Autodesk Inventor part; units mm, degrees
ref_plane "ROD_BA_XY" through (8, 0, 0) normal (-1, 0, 0) x (0, 0, -1)
ref_plane "ROD_BA_YZ" through (8, 0, 0) normal (0, 0, -1) x (0, -1, 0)
ref_plane "ROD_BA_ZX" through (8, 0, 0) normal (0, -1, 0) x (-1, 0, 0)
sketch "Sketch_2" plane through (0, 0, 0) normal (0, 0, 1) x (1, 0, 0)
  line L0 (75.5, 0) -> (0, 0)
  line L1 (0, 0) -> (0, 1.5705)
  line L2 (0, 1.5705) -> (0.4295, 2)
  line L3 (0.4295, 2) -> (15, 2)
  line L4 (15, 2) -> (15, 1.65)
  line L5 (15, 1.65) -> (16.5, 1.65)
  line L6 (16.5, 1.65) -> (16.5, 2)
  line L7 (16.5, 2) -> (70.5, 2)
  line L8 (70.5, 2) -> (70.5, 5)
  line L9 (70.5, 5) -> (75.5, 5)
  line L10 (75.5, 5) -> (75.5, 0)
  line L11 (75.5, 0) -> (0, 0)
revolve "Revolution1" add sketch "Sketch_2" angle 360 about axis through (75.5, 0, 0) along (1, 0, 0)
thread "Thread1"
ref_plane "ROD_BA_XY" through (8, 0, 0) normal (-1, 0, 0) x (0, 0, -1)
ref_plane "ROD_BA_YZ" through (8, 0, 0) normal (0, 0, -1) x (0, -1, 0)
ref_plane "ROD_BA_ZX" through (8, 0, 0) normal (0, -1, 0) x (-1, 0, 0)
ref_plane "ROD_BODY_XY" through (28, 0, 0) normal (1, 0, 0) x (0, 0, -1)
ref_plane "ROD_BODY_YZ" through (28, 0, 0) normal (0, 0, -1) x (0, 1, 0)
ref_plane "ROD_BODY_ZX" through (28, 0, 0) normal (0, 1, 0) x (1, 0, 0)
ref_plane "rodnt1_XY" through (7.5, 0, 0) normal (1, 0, 0) x (0, 0, -1)
ref_plane "rodnt1_YZ" through (7.5, 0, 0) normal (0, 0, -1) x (0, 1, 0)
ref_plane "rodnt1_ZX" through (7.5, 0, 0) normal (0, 1, 0) x (1, 0, 0)
properties part number "CJ2D10-30Z_ROD"
Can you work these out from the model? Positions are in its coordinate system, mm. A direction names the side the tool comes from. Coordinates: 2 decimals unless noted, no trailing zeros. Order: outer loops, then holes, each group sorted by start corner. A loop starts at its lowest first (then second) coordinate and runs counter-clockwise, first axis right, second up. Notation, with made-up numbers: (-14, 48.25) - (2, 48.25) arc R21 cw to (2, 79.25) - close; hole circle Ø10 at (75, 55). An arc over 180 degrees is marked (long way). Answer in a Markdown table with one row per item.
1. If we mould it in two halves opening along X, with no side actions, what happens to faces 1 (the flat face through (75.5, 0, 0)), 2 (the flat face through (70.5, 2.2, 0.1)), 3 (the cylindrical face through (44, 0, -2)), 4 (the cylindrical face through (15.76, -1.216, 1.115))? For each: pulls with the +X half, pulls with the -X half, needs draft (parallel to the pull), parting line crosses it, or undercut.
Reply:
| item | result |
|---|---|
| face 1 | pulls with the +X half |
| face 2 | pulls with the -X half |
| face 3 | needs draft |
| face 4 | undercut |
2. For faces 5 (the cylindrical face through (8, 0, -2)), 6 (the flat face through (0, 0, 0)), which set-ups out of +Z, -Z, +X, -X, +Y, -Y let a thin tool reach every point of the face, with its end or its side?
Reply:
| item | result |
|---|---|
| face 5 | -X |
| face 6 | +Z, -Z, -X, +Y, -Y |
3. Suppose I cut it at D-D (z = 3.25). Please give me the cut outline in (x, y), and give its area (3 significant figures).
Reply:
| item | result |
|---|---|
| outline | (70.5, -3.8) - (75.5, -3.8) - (75.5, 3.8) - (70.5, 3.8) - close |
| area | 38.0 mm^2 |
4. For pin 1 (2 mm diameter, centred on x = 34.5, y = 2, fed in from +Z); pin 2 (1.5 mm diameter, centred on x = 22.5, y = -2.5, fed in from +Z); pin 3 (1.5 mm diameter, centred on x = 19, y = 0.5, fed in from -Z), each with a flat end and sliding along its axis, tell me the tip position at first contact or that it passes through.
Reply:
| item | result |
|---|---|
| pin 1 | stops at z = 1.73 |
| pin 2 | stops at z = 0.97 |
| pin 3 | stops at z = -2 |
5. Suppose I cut it at A-A (z = 0). Please give me the cut outline in (x, y).
Reply:
| item | result |
|---|---|
| outline | (0, -1.57) - (0.43, -2) - (15, -2) - (15, -1.65) - (16.5, -1.65) - (16.5, -2) - (70.5, -2) - (70.5, -5) - (75.5, -5) - (75.5, 5) - (70.5, 5) - (70.5, 2) - (16.5, 2) - (16.5, 1.65) - (15, 1.65) - (15, 2) - (0.43, 2) - (0, 1.57) - close |
6. If I drill on line 1 along X through (y, z) = (-0.5, -4.25); line 2 along Y through (x, z) = (5, 0.25), over which ranges is the centre line in solid material (lowest first)?
Reply:
| item | result |
|---|---|
| line 1 | x = 70.5 to 75.5 |
| line 2 | y = -1.98 to 1.98 |
7. Suppose I cut it at C-C (x = 37). Please give me the cut outline in (y, z).
Reply:
| item | result |
|---|---|
| outline | circle Ø4 at (0, 0) |
